Autodesk Inventor part; units mm, degrees
ref_plane "YZ Plane" through (0, 0, 0) normal (1, 0, 0) x (0, 1, 0)
ref_plane "XZ Plane" through (0, 0, 0) normal (0, 1, 0) x (-1, 0, 0)
ref_plane "XY Plane" through (0, 0, 0) normal (0, 0, 1) x (1, 0, 0)
sketch "Sketch1" plane through (0, 0, 0) normal (0, 0, 1) x (1, 0, 0)
  line L0 (-20, 10) -> (20, 10)
  line L1 (20, 10) -> (20, -10)
  line L2 (20, -10) -> (-20, -10)
  line L3 (-20, -10) -> (-20, 10)
  line L4 (-20, 10) -> (20, -10) construction
  line L5 (20, 10) -> (-20, -10) construction
  line L6 (20, 0) -> (30, 0)
  line L7 (35, -35) -> (-35, -35)
  line L8 (-35, -35) -> (-35, 35)
  line L9 (-35, 35) -> (35, 35)
  line L10 (35, 35) -> (35, -35)
  line L11 (35, -35) -> (-35, 35) construction
  line L12 (-35, -35) -> (35, 35) construction
  line L13 (30, -30) -> (-30, 30) construction
  line L14 (-30, -30) -> (30, 30) construction
  circle A0 centre (-30, 30) radius 1.5
  circle A1 centre (30, 30) radius 1.5
  circle A2 centre (-30, -30) radius 1.5
  circle A3 centre (30, -30) radius 1.5
  line L15 (0, 10) -> (0, 20)
  line L16 (0, -10) -> (0, -20)
  circle A4 centre (0, 20) radius 1.5
  circle A5 centre (0, -20) radius 1.5
  point P0 (0, 0)
  dimension "d0" = 40
  dimension "d1" = 20
  dimension "d2" = 10
  dimension "d3" = 70
  dimension "d4" = 70
  dimension "d9" = 3
  dimension "d10" = 3
  dimension "d11" = 3
  dimension "d12" = 3
  dimension "d15" = 10
  dimension "d16" = 10
  dimension "d17" = 3
  dimension "d18" = 3
extrude "Extrusion3" add sketch "Sketch1" along normal blind 3
properties part number "Servo Holder TOP"
Geometry: final body of the model. Coordinates: model frame, mm. A direction names the side the tool comes from. Give positions to 0.01 mm unless a question says otherwise; leave off trailing zeros. Write each loop counter-clockwise with the first axis right and the second up, starting at its lowest first coordinate (ties: lowest second). Pieces come first, ordered by that corner, then holes.
1. Draft query along Y for faces 3 (the cylindrical face through (28.89, 28.99, 1.48)), 4 (the flat face through (0, 16, 3)), 5 (the flat face through (0, -35, 1)), 6 (the flat face through (0, 35, 1)). Return one class per face: released by +Y, released by -Y, zero draft, split by the parting line, or undercut.
2. Line query: probe 1 along Y at (x, z) = (-30, 1.9); probe 2 along Y at (x, z) = (0, 1.35); probe 3 along X at (y, z) = (-20, 1.8). Output: solid intervals per line, ascending.
3. Section query C-C, the plane y = 30. Return loops of the section in (x, z).
4. Section query A-A, the plane y = 1. Return loops of the section in (x, z), then the cut area to 3 significant figures.
5. Reachability of faces 1 (the flat face through (0, 16, 0)), 2 (the flat face through (0, -10, 1)) from +Z, -Z, +X, -X, +Y, -Y: full face, straight path, thin tool, end or side. Return the list, or none.
6. Section query B-B, the plane x = 0. Return loops of the section in (y, z), then the cut area to 3 significant figures.
7. Pin query (flat end, axial travel): P1, Ø3.5, axis at x = 0, y = -20, coming from the +Z side. Return the tip coordinate at first contact, or that it passes through.
Computed:
1. face 3: undercut
1. face 4: zero draft
1. face 5: released by -Y
1. face 6: released by +Y
2. probe 1: y = -35 to -31.5, -28.5 to 28.5, 31.5 to 35
2. probe 2: y = -35 to -21.5, -18.5 to -10, 10 to 18.5, 21.5 to 35
2. probe 3: x = -35 to -1.5, 1.5 to 35
3. outline: (-35, 0) - (-31.5, 0) - (-31.5, 3) - (-35, 3) - close; (-28.5, 0) - (28.5, 0) - (28.5, 3) - (-28.5, 3) - close; (31.5, 0) - (35, 0) - (35, 3) - (31.5, 3) - close
4. outline: (-35, 0) - (-20, 0) - (-20, 3) - (-35, 3) - close; (20, 0) - (35, 0) - (35, 3) - (20, 3) - close
4. area: 90.0 mm2
5. face 1: -Z, +X, -X, +Y, -Y
5. face 2: +Z, -Z
6. outline: (-35, 0) - (-21.5, 0) - (-21.5, 3) - (-35, 3) - close; (-18.5, 0) - (-10, 0) - (-10, 3) - (-18.5, 3) - close; (10, 0) - (18.5, 0) - (18.5, 3) - (10, 3) - close; (21.5, 0) - (35, 0) - (35, 3) - (21.5, 3) - close
6. area: 132 mm2
7. P1: stops at z = 3
